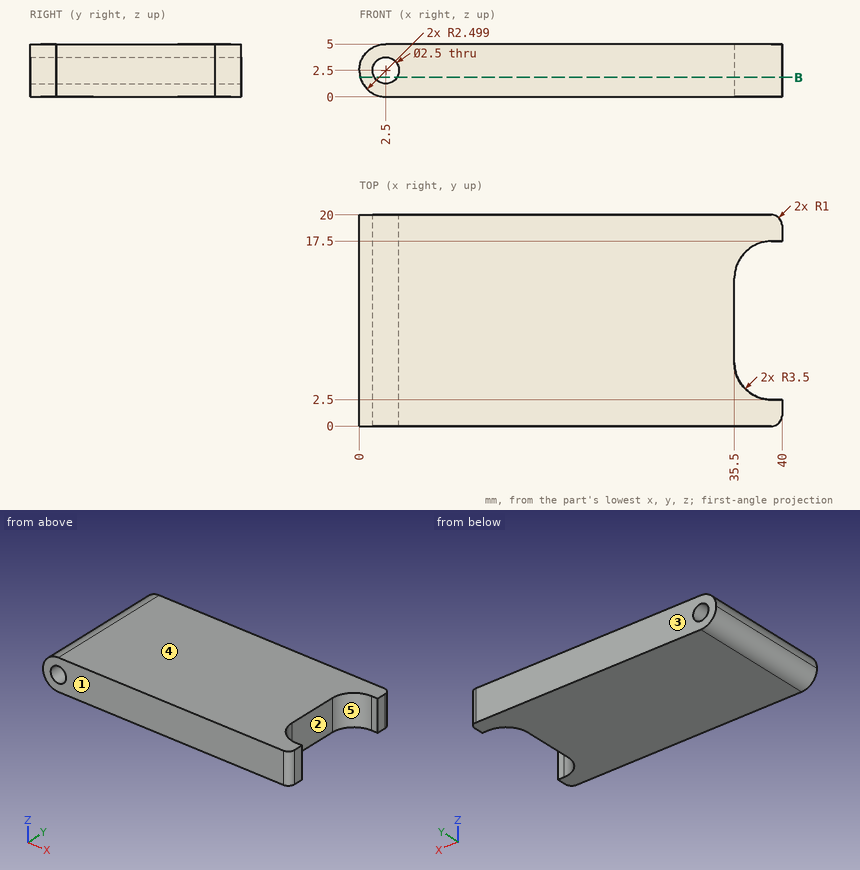
Can you work these out from the drawing? Everything is in mm from the part's minimum corner. A direction names the side the tool comes from. Give positions to 0.01 mm unless a question says otherwise; leave off trailing zeros. Order: outer loops, then holes, each group sorted by start corner. A loop starts at its lowest first (then second) coordinate and runs counter-clockwise, first axis right, second up. Notation, with made-up numbers: M 48,69 L 64,69 A19 cw 64,93 Z; hole C 61,-38.5 d8. An arc over 180 degrees is marked long. Write item = value, one per line. Start each with the question number.
Q1. For the marked faces 1 and 2, which set-ups out of +Z, -Z, +X, -X, +Y, -Y let a thin tool reach every point of the face, with its end or its side?
Q2. I need wall thicknesses on probe 1 along Z at (x, y) = (2.5, 7.5); probe 2 along X at (y, z) = (12.25, 2.5); probe 3 along X at (y, z) = (1, 4.5). Which ranges of each line are inside material? Lowest first, please. Write a range as [from, to].
Q3. We'd pull the mould along Y, two halves only. Please class the marked faces 3, 4 and 5: pulls with the +Y half, pulls with the -Y half, needs draft (parallel to the pull), parting line crosses it, or undercut.
Q4. Suppose I cut it at B-B (z = 1.85). Write out the boundary of the cut face in (x, y) (1 decimal).
Q5. Will these pins go through, and if not, where does the flat tip stop? pin 1 Ø0.5 at (x, z) = (39.5, 1.5) entering from +Y; pin 2 Ø3 at (y, z) = (6, 0.5) entering from +X; pin 3 Ø0.5 at (x, z) = (39.5, 3) entering from -Y; pin 4 Ø2 at (x, z) = (2.5, 2.5) entering from +Y.
Check result:
q1.face_1 = +Z, -Z, +X, -X, -Y
q1.face_2 = +Z, -Z, +X
q2.probe_1 = [0, 1.25], [3.75, 5]
q2.probe_2 = [0, 1.25], [3.75, 35.5]
q2.probe_3 = [1, 40]
q3.face_3 = pulls with the +Y half
q3.face_4 = needs draft
q3.face_5 = undercut
q4.outline = M 0.1,0 L 1.4,0 L 1.4,20 L 0.1,20 Z; M 3.6,0 L 39,0 A1 ccw 40,1 L 40,2.5 L 39,2.5 A3.5 cw 35.5,6 L 35.5,14 A3.5 cw 39,17.5 L 40,17.5 L 40,19 A1 ccw 39,20 L 3.6,20 Z
q5.pin_1 = 19.97
q5.pin_2 = 35.84
q5.pin_3 = 0.03
q5.pin_4 = through
